```python
from build123d import *

# Parameters (mm, degrees)
F2_DEPTH      = 2.5
F2_DEPTH_BACK = 2.5
F4_R          = 1


with BuildPart() as f2:
    # F1 (on offset) → F2 (new body, two sides)
    with BuildSketch(Plane.XY.offset(44)) as f2_sk:
        Polygon((-20.9, 0), (-16.9, 0), (-16.9, 6), (0, 11.1249185786), (-2.7934713079, 14.6528808873), (-18.9273972603, 9.7602739726), (-19.9136986301, 8.6301369863), (-20.9, 7.5), align=None)
    extrude(amount=F2_DEPTH)
    extrude(f2_sk.sketch, amount=-F2_DEPTH_BACK)

    # F3: F2 across plane


with BuildPart() as f2_1:
    add(f2.part)
    add(f2.part.mirror(Plane.XZ))

    # F4
    f4_edges = [f2_1.edges().sort_by_distance(p)[0] for p in [
        (-16.9, 0, 46.5),
        (-8.45, 8.562459, 46.5),
        (-1.396736, 12.8889, 46.5),
        (-10.860434, 12.206577, 46.5),
        (-19.913699, 8.630137, 46.5),
        (-20.9, 0, 46.5),
        (-19.913699, -8.630137, 46.5),
        (-10.860434, -12.206577, 46.5),
        (-1.396736, -12.8889, 46.5),
        (-8.45, -8.562459, 46.5),
        (-16.9, 0, 41.5),
        (-8.45, 8.562459, 41.5),
        (-1.396736, 12.8889, 41.5),
        (-10.860434, 12.206577, 41.5),
        (-19.913699, 8.630137, 41.5),
        (-20.9, 0, 41.5),
        (-19.913699, -8.630137, 41.5),
        (-10.860434, -12.206577, 41.5),
        (-1.396736, -12.8889, 41.5),
        (-8.45, -8.562459, 41.5),
    ]]
    fillet(f4_edges, radius=F4_R)


solid = f2_1.part
```
Model file for the job. Use its own axes, mm. A direction names the side the tool comes from. Give positions to 0.01 mm unless a question says otherwise; leave off trailing zeros. Order: outer loops, then holes, each group sorted by start corner. A loop starts at its lowest first (then second) coordinate and runs counter-clockwise, first axis right, second up.
1) 3-axis set-ups, long thin cutter, end or side, ignore diameter. For faces 5 (the flat face through (-10.75, 12.24, 44.02)), 6 (the flat face through (-8.568, 8.527, 44.021)), 7 (the flat face through (-18.3, -0.1, 46.5)), 8 (the cylindrical face through (-8.76, -8.77, 41.8)), 9 (the cylindrical face through (-8.76, 8.77, 46.2)): which of +Z, -Z, +X, -X, +Y, -Y reach the whole face in a straight line?
2) Saw through at A-A, the plane z = 44. Write the cut outline in (x, y), then the cut area to 3 significant figures.
3) Wall check: probe 1 along X at (y, z) = (3.25, 43.2); probe 2 along Y at (x, z) = (-12.75, 45.25); probe 3 along Y at (x, z) = (-1.5, 46.25). Give the ranges that are in metal, low to high.
4) Pin check, flat tips, straight feed: pin 1 (0.9 mm diameter, centred on y = 3, z = 44, fed in from +X); pin 2 (2 mm diameter, centred on x = -14, z = 43.5, fed in from -Y). Stop position of each tip, or through.
5) Mould opens along Y. For faces 1 (the cylindrical face through (-1.55, 12.81, 46.06)), 2 (the flat face through (-10.75, -12.24, 44.02)), 3 (the flat face through (-18.3, -0.1, 41.5)), 4 (the cylindrical face through (-17.185, -0.094, 41.801)) say: +Y half, -Y half, draft (parallel to the pull), parting line (faces both ways), or undercut.
6) Saw through at B-B, the plane y = 1.25. Write the cut outline in (x, z).
Computed:
1. face 5: +Z, -Z, -X, +Y
1. face 6: +Z, -Z, +X
1. face 7: +Z, +X, -X, +Y, -Y
1. face 8: -Z, +X
1. face 9: +Z, +X
2. outline: (-20.9, -7.5) - (-18.93, -9.76) - (-2.79, -14.65) - (0, -11.12) - (-16.9, -6) - (-16.9, 6) - (0, 11.12) - (-2.79, 14.65) - (-18.93, 9.76) - (-20.9, 7.5) - close
2. area: 211 mm2
3. probe 1: x = -20.9 to -16.9
3. probe 2: y = -11.63 to -7.26, 7.26 to 11.63
3. probe 3: y = -12.47 to -11.02, 11.02 to 12.47
4. pin 1: stops at x = -16.9
4. pin 2: stops at y = -11.56
5. face 1: +Y half
5. face 2: -Y half
5. face 3: draft
5. face 4: undercut
6. outline: (-20.9, 42.5) arc R1 ccw to (-19.9, 41.5) - (-17.9, 41.5) arc R1 ccw to (-16.9, 42.5) - (-16.9, 45.5) arc R1 ccw to (-17.9, 46.5) - (-19.9, 46.5) arc R1 ccw to (-20.9, 45.5) - close
